Study the drawing (mm; zero at the part's minimum x, y, z) and answer. Round coordinates to 2 decimals unless told otherwise and drop trailing zeros. Loops run counter-clockwise (first coordinate to the right, second up) from the corner with the lowest first, then second, coordinate; pieces in that order, holes last. Notation, with made-up numbers: M -25.5,45 L 17.5,45 A9 cw 17.5,59 Z; hole C 67,77 d11. An arc over 180 degrees is marked long. Put each result on its own line as item: value. Start each with the question number.
(1) Section C-C, the plane x = 28.99 is taken. Determine the outline of the cut face in (y, z) (1 decimal).
(2) Straight lines are drawn through the part: line 1 (Y direction, x = 15, z = 0.25) (1 decimal); line 2 (X direction, y = 7.5, z = 0.2); line 3 (Y direction, x = 4, z = 0.3) (1 decimal). For each, find the intervals that lie inside material, in ascending order.
(3) Section A-A, the plane x = 21 is taken. Determine the outline of the cut face in (y, z) (1 decimal).
(4) Section B-B, the plane z = 0.2 is taken. Count the separate pieces of the cut face and the enclosed holes in it, then the cut area to 3 significant figures.
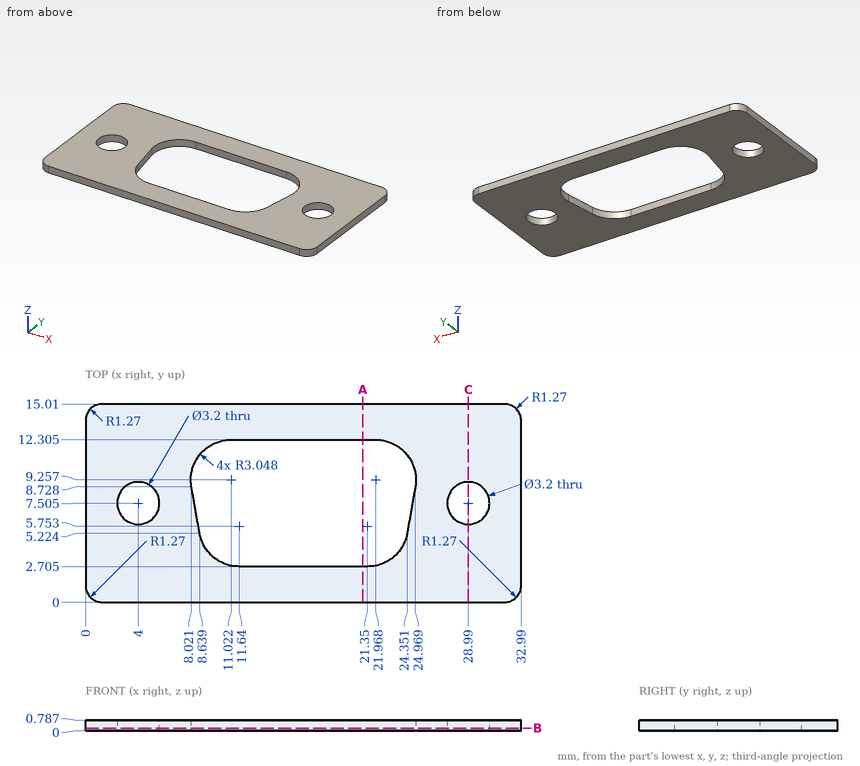
Recorded:
1. outline: M 0,0 L 5.9,0 L 5.9,0.8 L 0,0.8 Z; M 9.1,0 L 15,0 L 15,0.8 L 9.1,0.8 Z
2. line 1: y = 0 to 2.7, 12.3 to 15
2. line 2: x = 0 to 2.4, 5.6 to 8.24, 24.75 to 27.39, 30.59 to 32.99
2. line 3: y = 0 to 5.9, 9.1 to 15
3. outline: M 0,0 L 2.7,0 L 2.7,0.8 L 0,0.8 Z; M 12.3,0 L 15,0 L 15,0.8 L 12.3,0.8 Z
4. separate pieces: 1
4. enclosed holes: 3
4. area: 328 mm²
